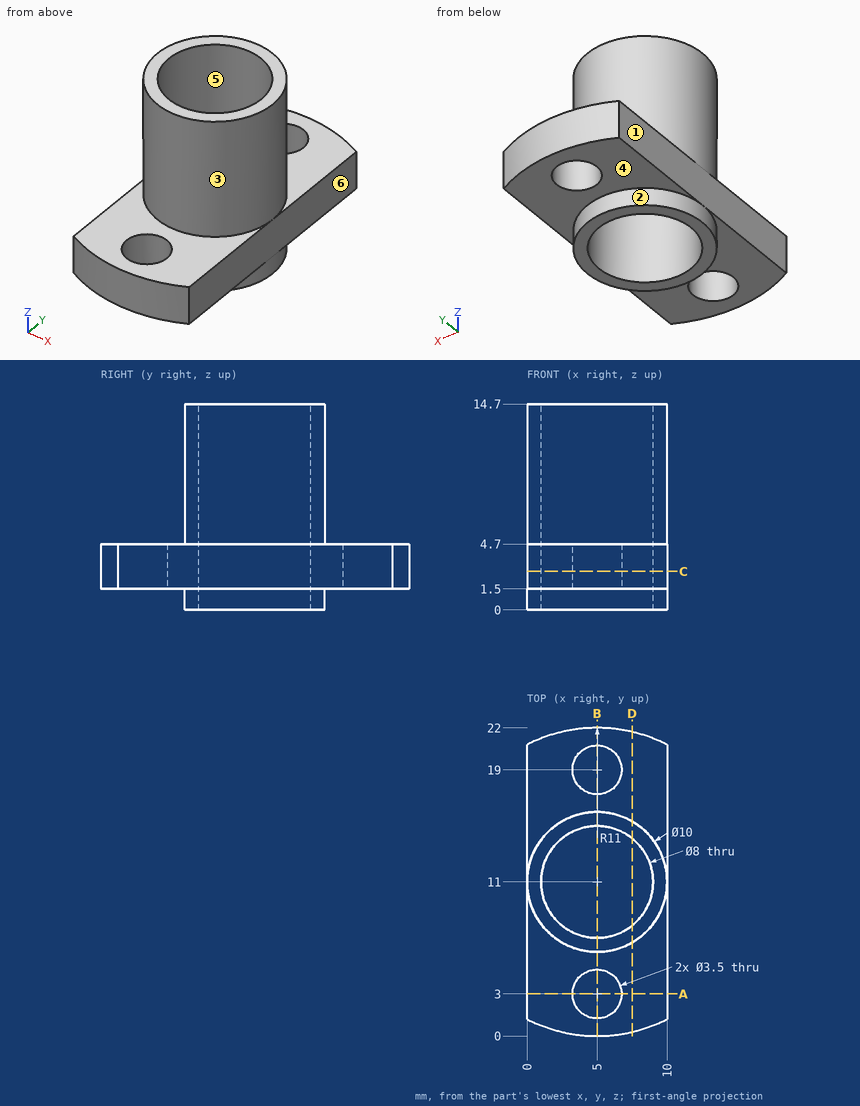
Could you check a few things on this drawing? It's one solid part, dimensions in mm from its lowest x, y, z. A direction names the side the tool comes from. Round coordinates to 2 decimals unless told otherwise and drop trailing zeros. Write each loop counter-clockwise with the first axis right and the second up, starting at its lowest first coordinate (ties: lowest second). Pieces come first, ordered by that corner, then holes. Notation, with made-up numbers: (64, 4.5) -> (95, 4.5) arc R6 ccw to (95, 13.5) -> close; hole circle Ø11 at (35.25, -19). An arc over 180 degrees is marked (long way). One line per item, written item: value.
1) For the marked faces 1, 2 and 3, which set-ups out of +Z, -Z, +X, -X, +Y, -Y let a thin tool reach every point of the face, with its end or its side?
Filled sheet:
face 1: +Z, -Z, -X, +Y, -Y
face 2: -Z
face 3: +Z
2) Suppose I cut it at D-D on x = 7.5. List the corners of the cut face in (y, z) for me.
Filled sheet:
outline: (0.29, 1.5) -> (6.67, 1.5) -> (6.67, 0) -> (7.88, 0) -> (7.88, 14.7) -> (6.67, 14.7) -> (6.67, 4.7) -> (0.29, 4.7) -> close; (14.12, 0) -> (15.33, 0) -> (15.33, 1.5) -> (21.71, 1.5) -> (21.71, 4.7) -> (15.33, 4.7) -> (15.33, 14.7) -> (14.12, 14.7) -> close
3) Suppose I cut it at A-A on y = 3. List the corners of the cut face in (x, z) for me, plus the area to 3 significant figures.
Filled sheet:
outline: (0, 1.5) -> (3.25, 1.5) -> (3.25, 4.7) -> (0, 4.7) -> close; (6.75, 1.5) -> (10, 1.5) -> (10, 4.7) -> (6.75, 4.7) -> close
area: 20.8 mm2
4) I'm going to push flat-ended pins straight in: pin 1 Ø2 at (x, z) = (1.5, 7.5) entering from +Y; pin 2 Ø1 at (x, z) = (9, 3) entering from -Y; pin 3 Ø4 at (x, y) = (5, 19) entering from +Z; pin 4 Ø1 at (x, y) = (2.5, 9.5) entering from +Z. Where does each tip first touch, or does it pass through?
Filled sheet:
pin 1: stops at y = 15.33
pin 2: stops at y = 0.57
pin 3: stops at z = 4.7
pin 4: passes through
5) If I drill on line 1 (Y direction, x = 5, z = 11.25); line 2 (Y direction, x = 6.5, z = 2); line 3 (Z direction, x = 0.5, y = 19.5), over which ranges is the centre line in solid material (lowest first)? Write a range as [from, to].
Filled sheet:
line 1: y = [6, 7], [15, 16]
line 2: y = [0.1, 2.1], [3.9, 7.29], [14.71, 18.1], [19.9, 21.9]
line 3: z = [1.5, 4.7]
6) We'd pull the mould along X, two halves only. Please class the marked faces 4, 5 and 6: released by +X, released by -X, zero draft, split by the parting line, or undercut.
Filled sheet:
face 4: zero draft
face 5: undercut
face 6: released by +X
7) Suppose I cut it at C-C on z = 2.75. List the corners of the cut face in (x, y) for me, plus the area to 3 significant figures.
Filled sheet:
outline: (0, 1.2) arc R11 ccw to (10, 1.2) -> (10, 20.8) arc R11 ccw to (0, 20.8) -> close; hole circle Ø8 at (5, 11); hole circle Ø3.5 at (5, 3); hole circle Ø3.5 at (5, 19)
area: 143 mm2
8) Suppose I cut it at B-B on x = 5. List the corners of the cut face in (y, z) for me.
Filled sheet:
outline: (0, 1.5) -> (1.25, 1.5) -> (1.25, 4.7) -> (0, 4.7) -> close; (4.75, 1.5) -> (6, 1.5) -> (6, 0) -> (7, 0) -> (7, 14.7) -> (6, 14.7) -> (6, 4.7) -> (4.75, 4.7) -> close; (15, 0) -> (16, 0) -> (16, 1.5) -> (17.25, 1.5) -> (17.25, 4.7) -> (16, 4.7) -> (16, 14.7) -> (15, 14.7) -> close; (20.75, 1.5) -> (22, 1.5) -> (22, 4.7) -> (20.75, 4.7) -> close
